Source: CAD feature listing. Evaluate the final solid. Frame: model axes, mm. Face numbers are marked on the shaded views. Give positions to 0.01 mm unless a question says otherwise; leave off trailing zeros. Write each loop counter-clockwise with the first axis right and the second up, starting at its lowest first coordinate (ties: lowest second). Pieces come first, ordered by that corner, then holes. Notation, with made-up numbers: M 86,-29.75 L 112,-29.75 A38 cw 112,9.25 Z; hole C 2,-3.5 d10. An arc over 180 degrees is marked long. Return JSON: item names as keys, results as strings.
```python
from build123d import *

# Parameters (mm, degrees)
F0_W            = 269
F0_H            = 32
F1_DEPTH        = 12
F2_W            = 217
F2_H            = 9
F2_H_2          = 11
F3_DEPTH        = 2
F5_D            = 2.4
F5_DEPTH        = 8
F5_TIP          = 0.7210327428
F7_D            = 4.1
F7_DEPTH        = 8
F7_TIP          = 1.231764269
F9_D            = 4.1
F9_DEPTH        = 8
F9_TIP          = 1.231764269
F11_D           = 4.1
F11_CBORE_D     = 9.75
F11_CBORE_DEPTH = 5


with BuildPart() as f1:
    # F0 (on Front) → F1 (new body)
    with BuildSketch(Plane.XZ):
        Rectangle(F0_W, F0_H)
    extrude(amount=F1_DEPTH)

    # F2 (on face) → F3 (join)
    with BuildSketch(Plane.XZ.offset(12)):
        with Locations((26, 11.5)):
            Rectangle(F2_W, F2_H)
        with Locations((26, -10.5)):
            Rectangle(F2_W, F2_H_2)
    extrude(amount=F3_DEPTH)

    # F5
    with Locations(Plane.XZ.offset(12)):
        with Locations((-33, 1), (-8, 1), (17, 1), (42, 1), (67, 1), (92, 1), (117, 1)):
            Hole(F5_D / 2, depth=F5_DEPTH)
            with Locations((0, 0, -(F5_DEPTH + F5_TIP / 2))):  # 118° drill point
                Cone(0, F5_D / 2, F5_TIP, mode=Mode.SUBTRACT)

    # F7
    with Locations(Plane.YZ.offset(134.5)):
        with Locations((-6, 10), (-6, -8)):
            Hole(F7_D / 2, depth=F7_DEPTH)
            with Locations((0, 0, -(F7_DEPTH + F7_TIP / 2))):  # 118° drill point
                Cone(0, F7_D / 2, F7_TIP, mode=Mode.SUBTRACT)

    # F9
    with Locations(Plane(origin=(-134.5, 0, 0), x_dir=(0, -1, 0), z_dir=(-1, 0, 0))):
        with Locations((6, 10), (6, -8)):
            Hole(F9_D / 2, depth=F9_DEPTH)
            with Locations((0, 0, -(F9_DEPTH + F9_TIP / 2))):  # 118° drill point
                Cone(0, F9_D / 2, F9_TIP, mode=Mode.SUBTRACT)

    # F11 (through all)
    with Locations(Plane.XY.offset(16)):
        with Locations((51.5, -6), (74.5, -6), (84.5, -6)):
            CounterBoreHole(F11_D / 2, F11_CBORE_D / 2, F11_CBORE_DEPTH)


solid = f1.part
```
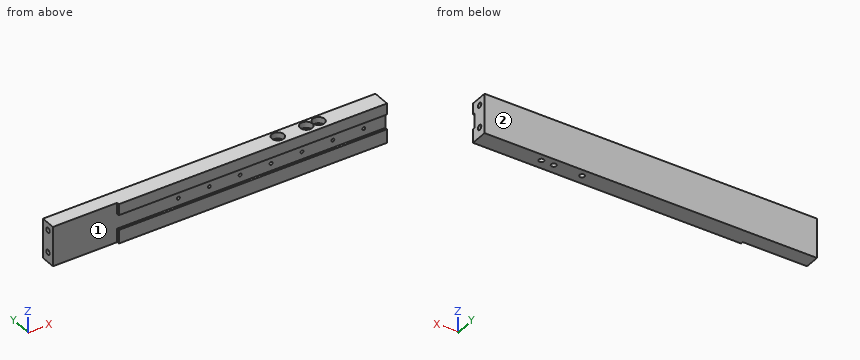
1) Contact query for flat-ended pins moving along their axis: pin 1 Ø2 at (x, z) = (67, 1) entering from -Y; pin 2 Ø3 at (y, z) = (-6, -7.5) entering from -X; pin 3 Ø1.5 at (x, z) = (-87, -3.5) entering from -Y. Output: stop coordinate, or through.
Numbers:
{"pin 1": "stops at y = -3.88", "pin 2": "stops at x = -126.47", "pin 3": "stops at y = -12"}
2) Line query: line 1 (Z direction, x = -129, y = -6); line 2 (X direction, y = -6.25, z = -12.5); line 3 (Y direction, x = -132, z = 10). Output: solid intervals per line, ascending. Write a range as [from, to].
Numbers:
{"line 1": "z = [-16, -10.05], [-5.95, 7.95], [12.05, 16]", "line 2": "x = [-134.5, 49.47], [53.53, 72.47], [76.53, 82.47], [86.53, 134.5]", "line 3": "y = [-12, -8.05], [-3.95, 0]"}
3) Cut plane A-A, the plane x = -3. Return the cut outline in (y, z).
Numbers:
{"outline": "M -14,-16 L 0,-16 L 0,16 L -14,16 L -14,7 L -12,7 L -12,-5 L -14,-5 Z"}
4) Draft query along Z for the marked faces 1 and 2. Return one class per face: released by +Z, released by -Z, zero draft, split by the parting line, or undercut.
Numbers:
{"face 1": "undercut", "face 2": "zero draft"}
5) Cut plane B-B, the plane x = -101.5. Return the cut outline in (y, z), then the cut area to 3 significant figures.
Numbers:
{"outline": "M -12,-16 L 0,-16 L 0,16 L -12,16 Z", "area": "384 mm²"}
